Geometry check sheet. Reference: drawing and pictorial views, mm from the part's lowest x, y, z. Coordinates: 2 decimals unless noted, no trailing zeros. Write each loop counter-clockwise with the first axis right and the second up, starting at its lowest first coordinate (ties: lowest second). Pieces come first, ordered by that corner, then holes. Notation, with made-up numbers: (24.25, 16) -> (53.25, 16) arc R15 ccw to (53.25, 40) -> close; hole circle Ø10 at (89.5, 32.25). An arc over 180 degrees is marked (long way). Put each result on its own line as item: value.
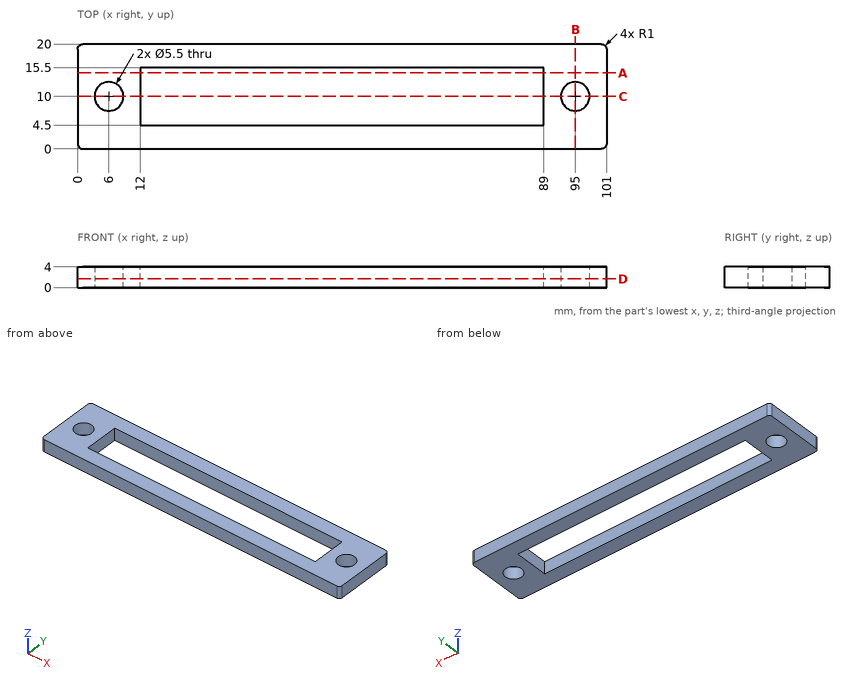
Q1. Cross-section at B-B (x = 95). Record the cut outline in (y, z), plus the area to 3 significant figures.
Recorded:
outline: (0, 0) -> (7.25, 0) -> (7.25, 4) -> (0, 4) -> close; (12.75, 0) -> (20, 0) -> (20, 4) -> (12.75, 4) -> close
area: 58.0 mm2
Q2. Cross-section at A-A (y = 14.5). Record the cut outline in (x, z), plus the area to 3 significant figures.
Recorded:
outline: (0, 0) -> (12, 0) -> (12, 4) -> (0, 4) -> close; (89, 0) -> (101, 0) -> (101, 4) -> (89, 4) -> close
area: 96.0 mm2
Q3. Cross-section at C-C (y = 10). Record the cut outline in (x, z), plus the area to 3 significant figures.
Recorded:
outline: (0, 0) -> (3.25, 0) -> (3.25, 4) -> (0, 4) -> close; (8.75, 0) -> (12, 0) -> (12, 4) -> (8.75, 4) -> close; (89, 0) -> (92.25, 0) -> (92.25, 4) -> (89, 4) -> close; (97.75, 0) -> (101, 0) -> (101, 4) -> (97.75, 4) -> close
area: 52.0 mm2
Q4. Depth check by flat-ended pin: P1, Ø10, axis at x = 75, y = 7.5, coming from the -Z side; P2, Ø4, axis at x = 19.5, y = 12.5, coming from the -Z side. Enter the tip coordinate at first touch or a pass-through.
Recorded:
P1: stops at z = 0
P2: passes through
Q5. Cross-section at D-D (z = 1.7). Record the cut outline in (x, y).
Recorded:
outline: (0, 1) arc R1 ccw to (1, 0) -> (100, 0) arc R1 ccw to (101, 1) -> (101, 19) arc R1 ccw to (100, 20) -> (1, 20) arc R1 ccw to (0, 19) -> close; hole circle Ø5.5 at (6, 10); hole (12, 4.5) -> (89, 4.5) -> (89, 15.5) -> (12, 15.5) -> close; hole circle Ø5.5 at (95, 10)
Q6. Material ranges on line 1 along X through (y, z) = (13.25, 1.95); line 2 along Y through (x, z) = (41.5, 1.75); line 3 along X through (y, z) = (7.75, 3.05), recorded low to high.
Recorded:
line 1: x = 0 to 12, 89 to 101
line 2: y = 0 to 4.5, 15.5 to 20
line 3: x = 0 to 4.42, 7.58 to 12, 89 to 93.42, 96.58 to 101
